Check sheet for the modelled part. Datum: model origin and axes. Units: mm. A direction names the side the tool comes from. Round coordinates to 2 decimals unless told otherwise and drop trailing zeros. Loops run counter-clockwise (first coordinate to the right, second up) from the corner with the lowest first, then second, coordinate; pieces in that order, holes last. Notation, with made-up numbers: (71, 26) -> (96, 26) arc R15 ccw to (96, 42) -> close; hole circle Ø6 at (-39, -36.75). An arc over 180 degrees is marked (long way). One line per item, written item: value. Start each with the question number.
1. Go/stop test with flat-tipped pins: pin 1 (5 mm diameter, centred on y = 1.5, z = -1.5, fed in from +X); pin 2 (2.5 mm diameter, centred on x = 2.5, z = 0, fed in from -Y); pin 3 (8 mm diameter, centred on x = 3, z = -3, fed in from -Y); pin 4 (1.3 mm diameter, centred on x = 10.5, y = 5.5, fed in from -Z). Record where each tip stops, or that it passes through.
2. Cross-section at B-B on y = 0. Record the cut outline in (x, z), then the cut area to 3 significant figures.
3. Cross-section at D-D on z = -4.75. Record the cut outline in (x, y).
4. Release check for a two-part mould opening along Y. For faces 1 (the face through (11, -5, 0)), 2 (the face through (2.465, -4.436, -2.307)), 3 (the face through (8.6, -5.61, -4.38)), 4 (the face through (7, 0, 0)) record: +Y half, -Y half, draft (parallel to the pull), parting line (faces both ways), or undercut.
5. Cross-section at A-A on x = 10.75. Record the cut outline in (y, z), then the cut area to 3 significant figures.
6. Cross-section at C-C on z = 0. Count the separate pieces of the cut face and the enclosed holes in it, then the cut area to 3 significant figures.
7. Set-up check for faces 5 (the face through (11, 5, 0)), 6 (the face through (5, -5, -2)), 7 (the face through (11, 6, -3.59)): record each of +Z, -Z, +X, -X, +Y, -Y from which the full face is reachable in a straight line by a thin tool's end or side.
8. Material ranges on L1, parallel to X at y = -6.8, z = 0; L2, parallel to X at y = -4, z = 0; L3, parallel to X at y = -1.75, z = -1.5, recorded low to high.
from build123d import *

# Parameters (mm, degrees)
SKETCH1_R               = 5
BOSS_EXTRUDE1_DEPTH     = 5
SKETCH2_R               = 7.5
BOSS_EXTRUDE2_DEPTH     = 2
BOSS_EXTRUDE3_DEPTH     = 10
CUT_EXTRUDE1_DEPTH      = 23.394195677
CUT_EXTRUDE1_DEPTH_BACK = 23.394195677
CUT_EXTRUDE2_DEPTH      = 23.092080194
CUT_EXTRUDE2_DEPTH_BACK = 23.092080194
SKETCH5_R               = 0.75
SKETCH6_R               = 2.5
CUT_EXTRUDE3_DEPTH      = 5
SKETCH7_R               = 1
CUT_EXTRUDE4_DEPTH      = 10


with BuildPart() as part:
    # Sketch1 → Boss-Extrude1 (new body)
    with BuildSketch(Plane(origin=(0, 0, 0), x_dir=(0, 0, -1), z_dir=(1, 0, 0))):
        Circle(SKETCH1_R)
    extrude(amount=BOSS_EXTRUDE1_DEPTH)

    # Sketch2 → Boss-Extrude2 (add)
    with BuildSketch(Plane(origin=(5, 0, 0), x_dir=(0, 0, -1), z_dir=(1, 0, 0))):
        Circle(SKETCH2_R)
    extrude(amount=BOSS_EXTRUDE2_DEPTH)

    # Sketch3 → Boss-Extrude3 (add)
    with BuildSketch(Plane(origin=(7, 0, 0), x_dir=(0, 0, -1), z_dir=(1, 0, 0))):
        with BuildLine():
            ThreePointArc((5.590169944, 5), (0, 7.5), (-5.590169944, 5))
            Line((-5.590169944, 5), (-4.898979486, 5))
            Line((-4.898979486, 5), (4.898979486, 5))
            Line((4.898979486, 5), (5.590169944, 5))
        make_face()
        with BuildLine():
            Line((-4.898979486, -5), (-5.590169944, -5))
            ThreePointArc((-5.590169944, -5), (0, -7.5), (5.590169944, -5))
            Line((5.590169944, -5), (4.898979486, -5))
            Line((4.898979486, -5), (-4.898979486, -5))
        make_face()
    extrude(amount=BOSS_EXTRUDE3_DEPTH)

    # Sketch4 → Cut-Extrude1 (cut, two sides: drawn at the far end of the back side and taken through both)
    with BuildSketch(Plane.XZ.offset(-5).offset(-CUT_EXTRUDE1_DEPTH_BACK)):
        with BuildLine():
            Line((7, 5.590169944), (17, 5.590169944))
            Line((17, 5.590169944), (17, -5.590169944))
            Line((17, -5.590169944), (7, -5.590169944))
            Line((7, -5.590169944), (9.640400827, -3.590169944))
            Line((9.640400827, -3.590169944), (12.640400827, -3.590169944))
            add(Edge.make_bspline(
                [(12.640400827, -3.590169944), (15.280133609, -2.393446629), (17.919866391, 0), (15.280133609, 2.393446629), (12.640400827, 3.590169944)],
                knots=[0.178885438, 0.178885438, 0.178885438, 0.178885438, 0.5, 0.821114562, 0.821114562, 0.821114562, 0.821114562], degree=3))
            Line((12.640400827, 3.590169944), (9.640400827, 3.590169944))
            Line((9.640400827, 3.590169944), (7, 5.590169944))
        make_face()
    extrude(amount=CUT_EXTRUDE1_DEPTH + CUT_EXTRUDE1_DEPTH_BACK, mode=Mode.SUBTRACT)

    # Sketch5 → Cut-Extrude2 (cut, two sides: drawn at the far end of the back side and taken through both)
    with BuildSketch(Plane.XZ.offset(-5).offset(-CUT_EXTRUDE2_DEPTH_BACK)):
        with Locations(Location((14, 0, 0), (0, 0, 270))):
            Circle(SKETCH5_R)
    extrude(amount=CUT_EXTRUDE2_DEPTH + CUT_EXTRUDE2_DEPTH_BACK, mode=Mode.SUBTRACT)

    # Sketch6 → Cut-Extrude3 (cut)
    with BuildSketch(Plane.ZY):
        Circle(SKETCH6_R)
    extrude(amount=-CUT_EXTRUDE3_DEPTH, mode=Mode.SUBTRACT)

    # Sketch7 → Cut-Extrude4 (cut, symmetric)
    with BuildSketch(Plane(origin=(0, 0, 0), x_dir=(1, 0, 0), z_dir=(0, 1, 0))):
        with Locations(Location((2.5, 0, 0), (0, 0, 270))):
            Circle(SKETCH7_R)
    extrude(amount=CUT_EXTRUDE4_DEPTH, both=True, mode=Mode.SUBTRACT)


solid = part.part
Taken from the geometry:
1. pin 1: stops at x = 7
1. pin 2: stops at y = -5
1. pin 3: stops at y = -7.5
1. pin 4: stops at z = -3.59
2. outline: (0, -5) -> (5, -5) -> (5, -7.5) -> (7, -7.5) -> (7, 7.5) -> (5, 7.5) -> (5, 5) -> (0, 5) -> (0, 2.5) -> (5, 2.5) -> (5, -2.5) -> (0, -2.5) -> close
2. area: 55.0 mm2
3. outline: (0, -1.56) -> (5, -1.56) -> (5, -5.8) -> (8.11, -5.8) -> (8.11, -5) -> (7, -5) -> (7, 5) -> (8.11, 5) -> (8.11, 5.8) -> (5, 5.8) -> (5, 1.56) -> (0, 1.56) -> close
4. face 1: undercut
4. face 2: parting line
4. face 3: draft
4. face 4: undercut
5. outline: (-6.58, -3.59) -> (-5, -3.59) -> (-5, 3.59) -> (-6.58, 3.59) arc R7.5 ccw to start; (5, -3.59) -> (6.58, -3.59) arc R7.5 ccw to (6.58, 3.59) -> (5, 3.59) -> close
5. area: 31.6 mm2
6. separate pieces: 5
6. enclosed holes: 0
6. area: 85.5 mm2
7. face 5: +Z, -Z, +X
7. face 6: -X
7. face 7: -Z, +X, +Y, -Y
8. L1: x = 5 to 13.25, 14.75 to 16.6
8. L2: x = 0 to 1.5, 3.5 to 7
8. L3: x = 5 to 7
